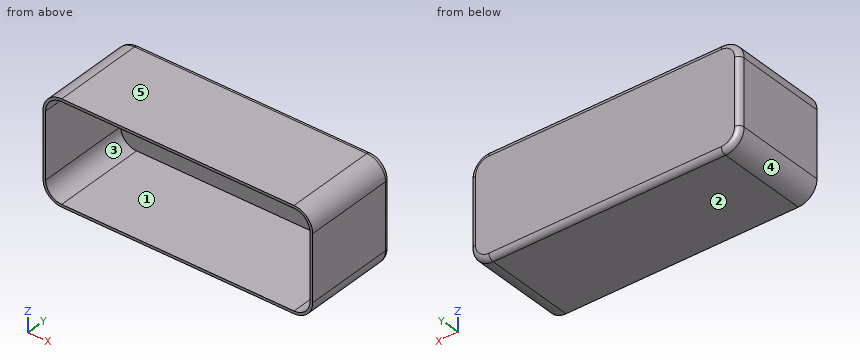
from build123d import *

# Parameters (mm, degrees)
BOSS_EXTRUDE1_DEPTH = 350
BOSS_EXTRUDE2_DEPTH = 10
FILLET1_R           = 20


with BuildPart() as part:
    # Sketch1 → Boss-Extrude1 (new body)
    with BuildSketch(Plane(origin=(0, 0, 0), x_dir=(1, 0, 0), z_dir=(0, 1, 0))):
        with BuildLine():
            Line((-505, -123), (-505, 123))
            ThreePointArc((-505, 123), (-484.497474683, 172.497474683), (-435, 193))
            Line((-435, 193), (435, 193))
            ThreePointArc((435, 193), (484.497474683, 172.497474683), (505, 123))
            Line((505, 123), (505, -123))
            ThreePointArc((505, -123), (484.497474683, -172.497474683), (435, -193))
            Line((435, -193), (-435, -193))
            ThreePointArc((-435, -193), (-484.497474683, -172.497474683), (-505, -123))
        make_face()
        with BuildLine():
            ThreePointArc((495, 123), (477.426406871, 165.426406871), (435, 183))
            Line((435, 183), (-435, 183))
            ThreePointArc((-435, 183), (-477.426406871, 165.426406871), (-495, 123))
            Line((-495, 123), (-495, -123))
            ThreePointArc((-495, -123), (-477.426406871, -165.426406871), (-435, -183))
            Line((-435, -183), (435, -183))
            ThreePointArc((435, -183), (477.426406871, -165.426406871), (495, -123))
            Line((495, -123), (495, 123))
        make_face(mode=Mode.SUBTRACT)
    extrude(amount=BOSS_EXTRUDE1_DEPTH)

    # Sketch2 → Boss-Extrude2 (add)
    with BuildSketch(Plane(origin=(0, 350, 0), x_dir=(1, 0, 0), z_dir=(0, 1, 0))):
        with BuildLine():
            Line((-435, -193), (435, -193))
            ThreePointArc((435, -193), (484.497474683, -172.497474683), (505, -123))
            Line((505, -123), (505, 123))
            ThreePointArc((505, 123), (484.497474683, 172.497474683), (435, 193))
            Line((435, 193), (-435, 193))
            ThreePointArc((-435, 193), (-484.497474683, 172.497474683), (-505, 123))
            Line((-505, 123), (-505, -123))
            ThreePointArc((-505, -123), (-484.497474683, -172.497474683), (-435, -193))
        make_face()
    extrude(amount=BOSS_EXTRUDE2_DEPTH)

    # Fillet1
    fillet1_edges = [part.edges().sort_by_distance(p)[0] for p in [
        (484.497474683, 360, -172.497474683),
        (0, 360, -193),
        (-484.497474683, 360, -172.497474683),
        (-505, 360, 0),
        (-484.497474683, 360, 172.497474683),
        (0, 360, 193),
        (484.497474683, 360, 172.497474683),
        (505, 360, 0),
    ]]
    fillet(fillet1_edges, radius=FILLET1_R)


solid = part.part
Part model, mm, in its own coordinate system. Face numbers are marked on the shaded views. A direction names the side the tool comes from. Give positions to 0.01 mm unless a question says otherwise; leave off trailing zeros. Loops run counter-clockwise (first coordinate to the right, second up) from the corner with the lowest first, then second, coordinate; pieces in that order, holes last. Notation, with made-up numbers: (63.5, 88) -> (78.5, 88) arc R28 cw to (78.5, 107) -> close; hole circle Ø9 at (-22, -15.5). An arc over 180 degrees is marked (long way). Write each question's results on one line, items separated by ' | '. Start each with the question number.
Q1. Pull direction Z, two halves, no side cores. Call the marked faces 3, 4 and 5: +Z half, -Z half, draft (parallel to the pull), parting line (faces both ways), or undercut.
Q2. Pin check, flat tips, straight feed: P1, Ø8, axis at y = 81.5, z = 126, coming from the +X side; P2, Ø4, axis at x = 85, z = -78.5, coming from the -Y side. Stop position of each tip, or through.
Q3. Band-saw the part on C-C on z = 41. List the corners of the cut face in (x, y).
Q4. Band-saw the part on B-B on x = -114. List the corners of the cut face in (y, z).
Q5. Which spindle directions (+Z, -Z, +X, -X, +Y, -Y) get a long thin tool onto all of the face, cutting with end or side? Do the marked faces 1 and 2. Say none if no direction does.
Q6. Wall check: L1, parallel to Z at x = 320, y = 176.5; L2, parallel to Z at x = -282, y = 342; L3, parallel to X at y = 97, z = -36. Give the ranges that are in metal, low to high.
Q7. Band-saw the part on A-A on y = 54.5. List the corners of the cut face in (x, z), plus the area to 3 significant figures.
Results are:
1) face 3: undercut | face 4: -Z half | face 5: +Z half
2) P1: stops at x = 505 | P2: stops at y = 350
3) outline: (-505, 0) -> (-495, 0) -> (-495, 350) -> (495, 350) -> (495, 0) -> (505, 0) -> (505, 340) arc R20 ccw to (485, 360) -> (-485, 360) arc R20 ccw to (-505, 340) -> close
4) outline: (0, -193) -> (340, -193) arc R20 ccw to (360, -173) -> (360, 173) arc R20 ccw to (340, 193) -> (0, 193) -> (0, 183) -> (350, 183) -> (350, -183) -> (0, -183) -> close
5) face 1: -Y | face 2: -Z, +X, -X, +Y, -Y
6) L1: z = -193 to -183, 183 to 193 | L2: z = -192.9 to -183, 183 to 192.9 | L3: x = -505 to -495, 495 to 505
7) outline: (-505, -123) arc R70 ccw to (-435, -193) -> (435, -193) arc R70 ccw to (505, -123) -> (505, 123) arc R70 ccw to (435, 193) -> (-435, 193) arc R70 ccw to (-505, 123) -> close; hole (-495, -123) arc R60 ccw to (-435, -183) -> (435, -183) arc R60 ccw to (495, -123) -> (495, 123) arc R60 ccw to (435, 183) -> (-435, 183) arc R60 ccw to (-495, 123) -> close | area: 26,400 mm²
